Source: CAD feature listing. Evaluate the final solid. Frame: model axes, mm. Coordinates: 2 decimals unless noted, no trailing zeros. Order: outer loops, then holes, each group sorted by start corner. A loop starts at its lowest first (then second) coordinate and runs counter-clockwise, first axis right, second up. Notation, with made-up numbers: (24.5, 58.5) - (67.5, 58.5) arc R20 cw to (67.5, 95.5) - close; hole circle Ø4 at (79.25, 31). An arc over 180 degrees is marked (long way). One line per question, with ' | ' between items. Start each with the question number.
(1) Section B-B (y = 8.5). Return the cut outline in (x, z), then the cut area to 3 significant figures.
(2) Contact query for flat-ended pins moving along their axis: P1, Ø12, axis at x = 321.5, y = 3, coming from the +Z side; P2, Ø8, axis at x = 708.66, z = -16.51, coming from the +Y side; P3, Ø6.5, axis at x = 64.5, y = 20.5, coming from the +Z side; P4, Ø12, axis at x = 361.5, z = -7, coming from the +Y side. Output: stop coordinate, or through.
(3) Line query: line 1 along X through (y, z) = (18.5, -3); line 2 along X through (y, z) = (20.25, -16.51); line 3 along X through (y, z) = (4.5, -7.62). Output: solid intervals per line, ascending.
(4) Section A-A (z = -7.62). Return the cut outline in (x, y), then the cut area to 3 significant figures.
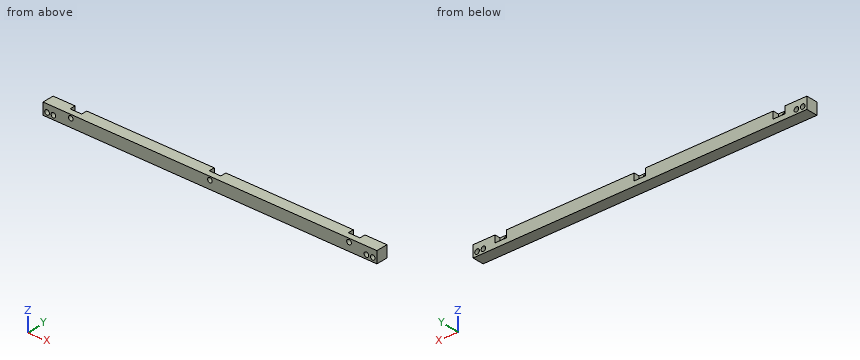
from build123d import *

# Parameters (mm, degrees)
SKETCH1_W           = 731.52
SKETCH1_H           = 25.4
BOSS_EXTRUDE1_DEPTH = 25.4
SKETCH2_R           = 5.08
CUT_EXTRUDE1_DEPTH  = 27.94
SKETCH3_W           = 25.4
SKETCH3_H           = 15.24
CUT_EXTRUDE2_DEPTH  = 12.7
SKETCH4_R           = 5.08
CUT_EXTRUDE3_DEPTH  = 15.24


with BuildPart() as part:
    # Sketch1 → Boss-Extrude1 (new body)
    with BuildSketch(Plane(origin=(0, 0, 0), x_dir=(1, 0, 0), z_dir=(0, 1, 0))):
        with Locations((365.76, 12.7)):
            Rectangle(SKETCH1_W, SKETCH1_H)
    extrude(amount=BOSS_EXTRUDE1_DEPTH)

    # Sketch2 → Cut-Extrude1 (cut)
    with BuildSketch(Plane(origin=(0, 25.4, 0), x_dir=(1, 0, 0), z_dir=(0, 1, 0))):
        with Locations(Location((8.89, 16.51, 0), (0, 0, 270))):
            Circle(SKETCH2_R)
        with Locations(Location((22.86, 16.51, 0), (0, 0, 270))):
            Circle(SKETCH2_R)
        with Locations(Location((722.63, 16.51, 0), (0, 0, 270))):
            Circle(SKETCH2_R)
        with Locations(Location((708.66, 16.51, 0), (0, 0, 270))):
            Circle(SKETCH2_R)
    extrude(amount=-CUT_EXTRUDE1_DEPTH, mode=Mode.SUBTRACT)

    # Sketch3 → Cut-Extrude2 (cut)
    with BuildSketch(Plane(origin=(0, 25.4, 0), x_dir=(1, 0, 0), z_dir=(0, 1, 0))):
        with Locations((60.96, 7.62)):
            Rectangle(SKETCH3_W, SKETCH3_H)
        with Locations((670.56, 7.62)):
            Rectangle(SKETCH3_W, SKETCH3_H)
        with Locations((365.76, 7.62)):
            Rectangle(SKETCH3_W, SKETCH3_H)
    extrude(amount=-CUT_EXTRUDE2_DEPTH, mode=Mode.SUBTRACT)

    # Sketch4 → Cut-Extrude3 (cut)
    with BuildSketch(Plane(origin=(0, 12.7, 0), x_dir=(1, 0, 0), z_dir=(0, 1, 0))):
        with Locations(Location((60.96, 7.62, 0), (0, 0, 270))):
            Circle(SKETCH4_R)
        with Locations(Location((670.56, 7.62, 0), (0, 0, 270))):
            Circle(SKETCH4_R)
        with Locations(Location((365.76, 7.62, 0), (0, 0, 270))):
            Circle(SKETCH4_R)
    extrude(amount=-CUT_EXTRUDE3_DEPTH, mode=Mode.SUBTRACT)


solid = part.part
Response values:
1) outline: (0, -25.4) - (731.52, -25.4) - (731.52, 0) - (0, 0) - close; hole circle Ø10.16 at (8.89, -16.51); hole circle Ø10.16 at (22.86, -16.51); hole circle Ø10.16 at (60.96, -7.62); hole circle Ø10.16 at (365.76, -7.62); hole circle Ø10.16 at (670.56, -7.62); hole circle Ø10.16 at (708.66, -16.51); hole circle Ø10.16 at (722.63, -16.51) | area: 18,000 mm²
2) P1: stops at z = 0 | P2: passes through | P3: stops at z = -15.24 | P4: stops at y = 12.7
3) line 1: x = 0 to 48.26, 73.66 to 353.06, 378.46 to 657.86, 683.26 to 731.52 | line 2: x = 0 to 3.81, 13.97 to 17.78, 27.94 to 703.58, 713.74 to 717.55, 727.71 to 731.52 | line 3: x = 0 to 55.88, 66.04 to 360.68, 370.84 to 665.48, 675.64 to 731.52
4) outline: (0, 0) - (55.88, 0) - (55.88, 12.7) - (48.26, 12.7) - (48.26, 25.4) - (0, 25.4) - close; (66.04, 0) - (360.68, 0) - (360.68, 12.7) - (353.06, 12.7) - (353.06, 25.4) - (73.66, 25.4) - (73.66, 12.7) - (66.04, 12.7) - close; (370.84, 0) - (665.48, 0) - (665.48, 12.7) - (657.86, 12.7) - (657.86, 25.4) - (378.46, 25.4) - (378.46, 12.7) - (370.84, 12.7) - close; (675.64, 0) - (731.52, 0) - (731.52, 25.4) - (683.26, 25.4) - (683.26, 12.7) - (675.64, 12.7) - close | area: 17,200 mm²
